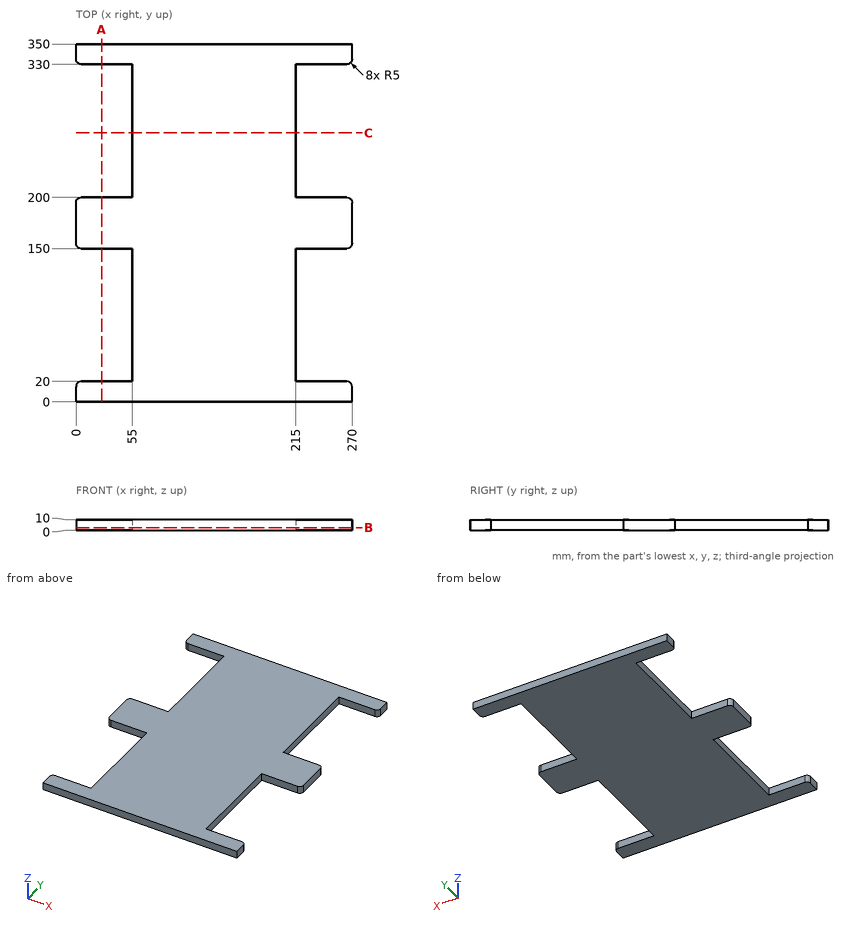
Source: three-view drawing plus pictorial views. Frame: mm from the lowest corner of the part. Give positions to 0.01 mm unless a question says otherwise; leave off trailing zeros. Order: outer loops, then holes, each group sorted by start corner. A loop starts at its lowest first (then second) coordinate and runs counter-clockwise, first axis right, second up. Notation, with made-up numbers: (26.5, 45) -> (30.5, 45) arc R30 ccw to (30.5, 71) -> close; hole circle Ø10 at (-23.75, 79). An arc over 180 degrees is marked (long way). Write each question's results on one line, items separated by ' | '. Start each with the question number.
Item 1: Cut plane B-B on z = 2.5. Return the cut outline in (x, y).
Item 2: Line query: line 1 (Y direction, x = 217, z = 8.5); line 2 (X direction, y = 327.5, z = 7.5). Output: solid intervals per line, ascending.
Item 3: Cut plane A-A on x = 25. Return the cut outline in (y, z), then the cut area to 3 significant figures.
Item 4: Cut plane C-C on y = 263. Return the cut outline in (x, z).
Item 5: Contact query for flat-ended pins moving along their axis: P1, Ø5, axis at y = 177.5, z = 2, coming from the -X side; P2, Ø4, axis at y = 292, z = 6, coming from the +X side; P3, Ø5, axis at y = 95.5, z = 6, coming from the -X side. Output: stop coordinate, or through.
Established:
1) outline: (0, 0) -> (270, 0) -> (270, 15) arc R5 ccw to (265, 20) -> (215, 20) -> (215, 150) -> (265, 150) arc R5 ccw to (270, 155) -> (270, 195) arc R5 ccw to (265, 200) -> (215, 200) -> (215, 330) -> (265, 330) arc R5 ccw to (270, 335) -> (270, 350) -> (0, 350) -> (0, 335) arc R5 ccw to (5, 330) -> (55, 330) -> (55, 200) -> (5, 200) arc R5 ccw to (0, 195) -> (0, 155) arc R5 ccw to (5, 150) -> (55, 150) -> (55, 20) -> (5, 20) arc R5 ccw to (0, 15) -> close
2) line 1: 0 to 20, 150 to 200, 330 to 350 | line 2: 55 to 215
3) outline: (0, 0) -> (20, 0) -> (20, 10) -> (0, 10) -> close; (150, 0) -> (200, 0) -> (200, 10) -> (150, 10) -> close; (330, 0) -> (350, 0) -> (350, 10) -> (330, 10) -> close | area: 900 mm^2
4) outline: (55, 0) -> (215, 0) -> (215, 10) -> (55, 10) -> close
5) P1: x = 0 | P2: x = 215 | P3: x = 55
